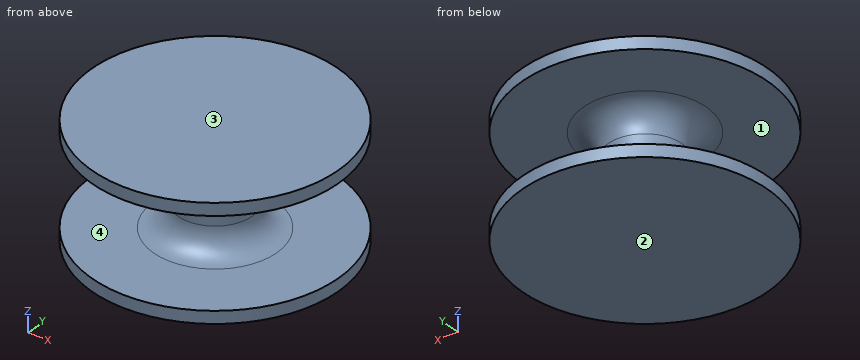
```python
from build123d import *

# Parameters (mm, degrees)
SKETCH7_R      = 5
EXTRUDE5_DEPTH = 2.30625
SKETCH8_W      = 3.5
SKETCH8_H      = 3.6125
FILLET1_R      = 1


with BuildPart() as part:
    # Sketch7 → Extrude5 (new body, symmetric)
    with BuildSketch(Plane.XY):
        Circle(SKETCH7_R)
    extrude(amount=EXTRUDE5_DEPTH, both=True)

    # Sketch8 → Cut-Revolve1 (revolve, cut)
    with BuildSketch(Plane(origin=(0, 0, 0), x_dir=(1, 0, 0), z_dir=(0, 1, 0)), mode=Mode.PRIVATE) as cut_revolve1_sk:
        with Locations((-3.25, 0)):
            Rectangle(SKETCH8_W, SKETCH8_H)
    revolve(cut_revolve1_sk.sketch.rotate(Axis((0, 0, 0), (0, 0, -1)), 180), axis=Axis((0, 0, 0), (0, 0, -1)), mode=Mode.SUBTRACT)  # turned: the seam where the file's is

    # Fillet1
    fillet1_edges = [part.edges().sort_by_distance(p)[0] for p in [
        (-1.5, 0, 1.80625),
        (-1.5, 0, -1.80625),
    ]]
    fillet(fillet1_edges, radius=FILLET1_R)


solid = part.part
```
Geometry check sheet. Reference: the model listing, model coordinates, mm. Face numbers are marked on the shaded views. Give positions to 0.01 mm unless a question says otherwise; leave off trailing zeros. Order: outer loops, then holes, each group sorted by start corner. A loop starts at its lowest first (then second) coordinate and runs counter-clockwise, first axis right, second up. Notation, with made-up numbers: (-27.5, 38) - (7.5, 38) arc R17 ccw to (7.5, 56) - close; hole circle Ø7 at (68.25, 55.5). An arc over 180 degrees is marked (long way). Write item = value, one per line. Start each with the question number.
1) Gauge pin test, flat end, axial feed: pin 1 Ø1 at (y, z) = (-1.5, -1) entering from +X. Record the tip position at first contact, or that the pin passes through.
2) Scan lines: L1, parallel to Z at x = -1.5, y = 2.5; L2, parallel to Z at x = -1.5, y = 1.25; L3, parallel to Y at x = 1, z = 1.85. Record each from-to range of solid material in increasing order.
3) Section check C-C (x = 0). Enter the section's corners in (y, z), then the cut area to 3 significant figures.
4) Section check A-A (x = -4). Enter the section's corners in (y, z), then the cut area to 3 significant figures.
5) Section check B-B (y = -4.5). Enter the section's corners in (x, z), then the cut area to 3 significant figures.
6) Draft check along Z on the marked faces 1, 2, 3 and 4. Enter one of: released by +Z, released by -Z, zero draft, split by the parting line, or undercut.
Geometry check:
q1.pin_1 = 1.21
q2.L1 = -2.31 to -1.81, 1.81 to 2.31
q2.L2 = -2.31 to -1.64, 1.64 to 2.31
q2.L3 = -4.9 to 4.9
q3.outline = (-5, -2.31) - (5, -2.31) - (5, -1.81) - (2.5, -1.81) arc R1 cw to (1.5, -0.81) - (1.5, 0.81) arc R1 cw to (2.5, 1.81) - (5, 1.81) - (5, 2.31) - (-5, 2.31) - (-5, 1.81) - (-2.5, 1.81) arc R1 cw to (-1.5, 0.81) - (-1.5, -0.81) arc R1 cw to (-2.5, -1.81) - (-5, -1.81) - close
q3.area = 21.7 mm2
q4.outline = (-3, -2.31) - (3, -2.31) - (3, -1.81) - (-3, -1.81) - close; (-3, 1.81) - (3, 1.81) - (3, 2.31) - (-3, 2.31) - close
q4.area = 6.00 mm2
q5.outline = (-2.18, -2.31) - (2.18, -2.31) - (2.18, -1.81) - (-2.18, -1.81) - close; (-2.18, 1.81) - (2.18, 1.81) - (2.18, 2.31) - (-2.18, 2.31) - close
q5.area = 4.36 mm2
q6.face_1 = undercut
q6.face_2 = released by -Z
q6.face_3 = released by +Z
q6.face_4 = undercut
